Verification items for the finished model (mm, model axes). Face numbers are marked on the shaded views. A direction names the side the tool comes from. Round coordinates to 2 decimals unless told otherwise and drop trailing zeros. Order: outer loops, then holes, each group sorted by start corner. A loop starts at its lowest first (then second) coordinate and runs counter-clockwise, first axis right, second up.
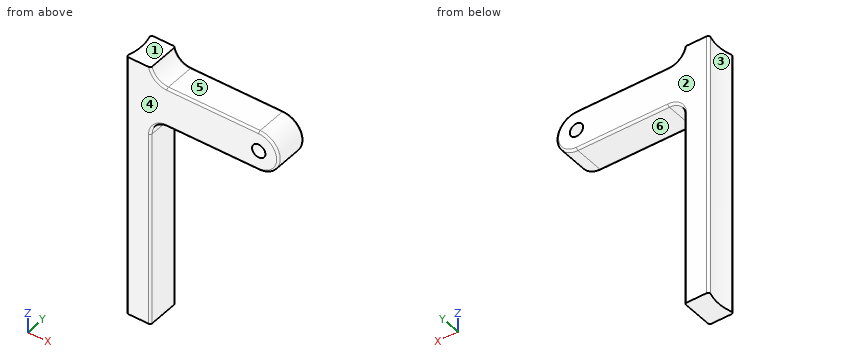
```python
from build123d import *

# Parameters (mm, degrees)
SKETCH1_R               = 1.27
BOSS_EXTRUDE1_DEPTH     = 3.175
FILLET1_R               = 3.175
CUT_EXTRUDE1_DEPTH      = 57.884801353
CUT_EXTRUDE1_DEPTH_BACK = 57.884801353
SKETCH3_R               = 8.89
FILLET2_R               = 0.396875


with BuildPart() as part:
    # Sketch1 → Boss-Extrude1 (new, symmetric)
    with BuildSketch(Plane(origin=(0, 0, 0), x_dir=(1, 0, 0), z_dir=(0, 1, 0))):
        with BuildLine():
            Line((-20.6375, -3.81), (-20.6375, -6.35))
            Line((-20.6375, -6.35), (-25.4, -6.35))
            Line((-25.4, -6.35), (-25.4, 44.45))
            Line((-25.4, 44.45), (-20.6375, 44.45))
            Line((-20.6375, 44.45), (-20.6375, 3.81))
            Line((-20.6375, 3.81), (0, 3.81))
            ThreePointArc((0, 3.81), (3.81, 0), (0, -3.81))
            Line((0, -3.81), (-20.6375, -3.81))
        make_face()
        with Locations(Location((0, 0, 0), (0, 0, 270))):
            Circle(SKETCH1_R, mode=Mode.SUBTRACT)
    extrude(amount=BOSS_EXTRUDE1_DEPTH, both=True)

    # Fillet1
    # the kernel refuses this fillet: 3.175 mm, written as the material it adds along each edge
    with BuildSketch(Plane(origin=(-20.6375, 3.175, 3.81), x_dir=(1, 0, 0), z_dir=(0, -1, 0))) as fillet1_piece_1:
        with BuildLine():
            CenterArc((3.110851973, 3.175), FILLET1_R, 191.536959033, 78.463040967)
            Line((0, 2.54), (-0.062217039, 2.5273))
            ThreePointArc((-0.062217039, 2.5273), (-0.0635, 1.27), (-0.0635, 0))
            Line((-0.0635, 0), (0, -0.0635))
            Line((0, -0.0635), (3.110851973, -0.0635))
            Line((3.110851973, -0.0635), (3.110851973, 0))
        make_face()
    extrude(amount=6.35)
    with BuildSketch(Plane(origin=(-20.6375, -3.175, -3.81), x_dir=(1, 0, 0), z_dir=(0, 1, 0))) as fillet1_piece_2:
        with BuildLine():
            CenterArc((FILLET1_R, FILLET1_R), FILLET1_R, 180, 90)
            Line((0, FILLET1_R), (-FILLET1_R * 0.02, FILLET1_R))
            Line((-FILLET1_R * 0.02, FILLET1_R), (-FILLET1_R * 0.02, -FILLET1_R * 0.02))
            Line((-FILLET1_R * 0.02, -FILLET1_R * 0.02), (FILLET1_R, -FILLET1_R * 0.02))
            Line((FILLET1_R, -FILLET1_R * 0.02), (FILLET1_R, 0))
        make_face()
    extrude(amount=6.35)

    # Sketch3 → Cut-Extrude1 (cut, two sides: drawn at the far end of the back side and taken through both)
    with BuildSketch(Plane.XY.offset(6.35).offset(-CUT_EXTRUDE1_DEPTH_BACK)):
        with Locations((-33.703702487, 0)):
            Circle(SKETCH3_R)
    extrude(amount=CUT_EXTRUDE1_DEPTH + CUT_EXTRUDE1_DEPTH_BACK, mode=Mode.SUBTRACT)

    # Fillet2
    fillet2_edges = [part.edges().sort_by_distance(p)[0] for p in [
        (-8.73125, -3.175, -3.81),
        (3.81, -3.175, 0),
        (-25.4, 3.175, -19.05),
        (-8.763324013, -3.175, 3.81),
        (-8.763324013, 3.175, 3.81),
        (-20.6375, -3.175, -25.7175),
        (-20.6375, 3.175, -25.7175),
        (-19.534694341, -3.175, 4.525655575),
        (-19.534694341, 3.175, 4.525655575),
        (-19.70756403, -3.175, -4.73993597),
        (-19.70756403, 3.175, -4.73993597),
        (3.81, 3.175, 0),
        (-8.73125, 3.175, -3.81),
        (-25.4, -3.175, -19.05),
    ]]
    fillet(fillet2_edges, radius=FILLET2_R)


solid = part.part
```
1) Draft check along Y on the marked faces 1, 2 and 3. Enter one of: released by +Y, released by -Y, zero draft, split by the parting line, or undercut.
2) Sectioned sample at A-A on z = 0. Record the cut outline in (x, y) (3 decimals).
3) Sectioned sample at D-D on x = -10. Record the cut outline in (y, z) (3 decimals).
4) Tool access check on the marked faces 4, 5 and 6. Record the directions out of +Z, -Z, +X, -X, +Y, -Y that give a thin tool (end or side, any length) a straight path to the whole face; none if there is none.
5) Go/stop test with flat-tipped pins: pin 1 Ø2 at (y, z) = (0, -19) entering from -X; pin 2 Ø3 at (x, y) = (-4.5, 1.5) entering from -Z; pin 3 Ø3 at (x, y) = (-8.5, -0.5) entering from +Z; pin 4 Ø1 at (x, z) = (-6.5, -5.5) entering from -Y. Record where each tip stops, or that it passes through.
6) Scan lines: probe 1 along X at (y, z) = (0.75, 0); probe 2 along X at (y, z) = (1.5, 0); probe 3 along Z at (x, y) = (-15, -1). Record each from-to range of solid material in increasing order.
7) Sectioned sample at C-C on z = -25. Record the cut outline in (x, y) (1 decimal), then the cut area to 3 significant figures.
Returned:
1. face 1: zero draft
1. face 2: released by +Y
1. face 3: undercut
2. outline: (-25.221, -2.659) arc R0.397 ccw to (-24.842, -3.175) - (-1.27, -3.175) - (-1.27, 3.175) - (-24.842, 3.175) arc R0.397 ccw to (-25.221, 2.659) arc R8.89 cw to start; (1.27, -3.175) - (3.413, -3.175) arc R0.397 ccw to (3.81, -2.778) - (3.81, 2.778) arc R0.397 ccw to (3.413, 3.175) - (1.27, 3.175) - close
3. outline: (-3.175, -3.413) arc R0.397 ccw to (-2.778, -3.81) - (2.778, -3.81) arc R0.397 ccw to (3.175, -3.413) - (3.175, 3.413) arc R0.397 ccw to (2.778, 3.81) - (-2.778, 3.81) arc R0.397 ccw to (-3.175, 3.413) - close
4. face 4: +Z, -Z, +X, -X, -Y
4. face 5: +Z, +X, +Y, -Y
4. face 6: -Z, +X, +Y, -Y
5. pin 1: stops at x = -24.87
5. pin 2: stops at z = -3.81
5. pin 3: stops at z = 3.81
5. pin 4: passes through
6. probe 1: x = -24.85 to -1.27, 1.27 to 3.81
6. probe 2: x = -24.94 to -1.27, 1.27 to 3.81
6. probe 3: z = -3.81 to 3.81
7. outline: (-25.2, -2.7) arc R0.4 ccw to (-24.8, -3.2) - (-21, -3.2) arc R0.4 ccw to (-20.6, -2.8) - (-20.6, 2.8) arc R0.4 ccw to (-21, 3.2) - (-24.8, 3.2) arc R0.4 ccw to (-25.2, 2.7) arc R8.9 cw to start
7. area: 27.5 mm2
